For this review, take the finished solid that the model builds, in its own axes (mm). A direction names the side the tool comes from. Give positions to 0.01 mm unless a question says otherwise; leave off trailing zeros. Order: outer loops, then holes, each group sorted by start corner. A loop starts at its lowest first (then second) coordinate and runs counter-clockwise, first axis right, second up.
Autodesk Inventor part; units mm, degrees
ref_plane "YZ Plane" through (0, 0, 0) normal (1, 0, 0) x (0, 1, 0)
ref_plane "XZ Plane" through (0, 0, 0) normal (0, 1, 0) x (-1, 0, 0)
ref_plane "XY Plane" through (0, 0, 0) normal (0, 0, 1) x (1, 0, 0)
sketch "Sketch1" plane through (0, 0, 0) normal (1, 0, 0) x (0, 1, 0)
  line L0 (43, 15.5) -> (-43, 15.5)
  line L1 (-43, 15.5) -> (-43, -15.5)
  line L2 (-43, -15.5) -> (43, -15.5)
  line L3 (43, -15.5) -> (43, 15.5)
  point P0 (0, 0)
  point P1 (0, -15.5)
  point P2 (43, 0)
  dimension "d0" = 86
  dimension "d1" = 31
extrude "Extrusion1" add sketch "Sketch1" along normal blind 5
sketch "Sketch2" plane through (5, 0, 0) normal (1, 0, 0) x (0, 0, -1)
  line L0 (-15.5, 43) -> (-12.5, 43)
  line L1 (-12.5, 43) -> (-12.5, -43)
  line L2 (-12.5, -43) -> (-15.5, -43)
  line L3 (-15.5, -43) -> (-15.5, 43)
  line L4 (12.5, 43) -> (15.5, 43)
  line L5 (15.5, 43) -> (15.5, -43)
  line L6 (15.5, -43) -> (12.5, -43)
  line L7 (12.5, -43) -> (12.5, 43)
  point P0 (0, 0)
  dimension "d4" = 3
  dimension "d5" = 3
extrude "Extrusion2" add sketch "Sketch2" along normal blind 12
sketch "Sketch3" plane through (0, -43, -15.5) normal (0, 0, -1) x (-1, 0, 0)
  line L0 (0, 86) -> (-17, 86) construction
  line L1 (-5, 0) -> (-5, 86) construction
  line L2 (-35.4485, 43) -> (35.4485, 43) construction
  line L3 (0, 0) -> (0, 86) construction
  point P0 (0, 43)
  point P1 (-13, 79.7)
  point P2 (0, 43)
  point P3 (-13, 6.3)
  dimension "d8" = 6.3
  dimension "d9" = 8
hole "Hole1" at (13, 36.7, -15.5) at (13, -36.7, -15.5) direction (0, 0, 1) diameter 4.8 end through all
sketch "Sketch4" plane through (5, 0, 0) normal (1, 0, 0) x (0, 0, -1)
  line L0 (-15.5, 43) -> (-15.5, -43)
  point P0 (0, 0)
  point P1 (-2.1, 10)
  dimension "d25" = 13.4
  dimension "d26" = 10
hole "Hole2" at (5, 10, 2.1) direction (-1, 0, 0) diameter 6.6 depth 5 counterbore diameter 11.4 counterbore depth 2.2
properties part number "TH_fan_holder"
1) Draft analysis for pull direction X (two halves, no side actions). For faces 1 (the face through (11, 1, 12.5)), 2 (the face through (12.28, -34.41, 14.02)), 3 (the face through (17, 1, 14)), 4 (the face through (12.894, 34.302, 14.021)), state which applies: +X half, -X half, draft (parallel to the pull), parting line (faces both ways), or undercut.
Answer sheet:
face 1: draft
face 2: undercut
face 3: +X half
face 4: undercut
2) To check wall thickness, follow line 1 (Y direction, x = 13, z = -13.7); line 2 (Z direction, x = 15, y = -24); line 3 (Z direction, x = 3.4, y = 10). State the ranges of each line that lie inside material, in increasing order.
Answer sheet:
line 1: y = -43 to -39.1, -34.3 to 34.3, 39.1 to 43
line 2: z = -15.5 to -12.5, 12.5 to 15.5
line 3: z = -15.5 to -3.6, 7.8 to 15.5
3) We need section D-D on y = 10. Give the boundary of the cut face in (x, z).
Answer sheet:
outline: (0, -15.5) - (17, -15.5) - (17, -12.5) - (5, -12.5) - (5, -3.6) - (2.8, -3.6) - (2.8, -1.2) - (0, -1.2) - close; (0, 5.4) - (2.8, 5.4) - (2.8, 7.8) - (5, 7.8) - (5, 12.5) - (17, 12.5) - (17, 15.5) - (0, 15.5) - close
4) We need section B-B on y = -36.7. Give the boundary of the cut face in (x, z).
Answer sheet:
outline: (0, -15.5) - (10.6, -15.5) - (10.6, -12.5) - (5, -12.5) - (5, 12.5) - (10.6, 12.5) - (10.6, 15.5) - (0, 15.5) - close; (15.4, -15.5) - (17, -15.5) - (17, -12.5) - (15.4, -12.5) - close; (15.4, 12.5) - (17, 12.5) - (17, 15.5) - (15.4, 15.5) - close
5) We need section A-A on x = 13. Give the boundary of the cut face in (y, z).
Answer sheet:
outline: (-43, -15.5) - (-39.1, -15.5) - (-39.1, -12.5) - (-43, -12.5) - close; (-43, 12.5) - (-39.1, 12.5) - (-39.1, 15.5) - (-43, 15.5) - close; (-34.3, -15.5) - (34.3, -15.5) - (34.3, -12.5) - (-34.3, -12.5) - close; (-34.3, 12.5) - (34.3, 12.5) - (34.3, 15.5) - (-34.3, 15.5) - close; (39.1, -15.5) - (43, -15.5) - (43, -12.5) - (39.1, -12.5) - close; (39.1, 12.5) - (43, 12.5) - (43, 15.5) - (39.1, 15.5) - close
6) Clearance check with a flat-ended pin moving along its axis: pin 1 (7.5 mm diameter, centred on y = 11, z = 6, fed in from +X). State where the tip first meets the part, or that it passes through.
Answer sheet:
pin 1: stops at x = 5
7) Tool access review of faces 5 (the face through (12.28, -34.41, -13.98)), 6 (the face through (3.88, 4.35, 2.84)), 7 (the face through (11, -1, -12.5)): name each direction out of +Z, -Z, +X, -X, +Y, -Y from which nothing blocks a thin tool from reaching the whole face with its end or side.
Answer sheet:
face 5: +Z, -Z
face 6: +X
face 7: +X, +Y, -Y
8) We need section C-C on z = 0.5. Give the boundary of the cut face in (x, y), then the cut area to 3 significant figures.
Answer sheet:
outline: (0, -43) - (5, -43) - (5, 4.53) - (2.8, 4.53) - (2.8, 7.11) - (0, 7.11) - close; (0, 12.89) - (2.8, 12.89) - (2.8, 15.47) - (5, 15.47) - (5, 43) - (0, 43) - close
area: 390 mm2
